Model file for the job. Use its own axes, mm. A direction names the side the tool comes from. Give positions to 0.01 mm unless a question says otherwise; leave off trailing zeros. Order: outer loops, then holes, each group sorted by start corner. A loop starts at its lowest first (then second) coordinate and runs counter-clockwise, first axis right, second up. Notation, with made-up numbers: (51, 9.5) - (75, 9.5) arc R26 ccw to (75, 40.5) - close; hole circle Ø4 at (68, 28.25). An arc over 180 degrees is marked (long way). Return JSON: item names as keys, results as strings. Group by question number.
from build123d import *

# Parameters (mm, degrees)
F0_W      = 50.8
F0_H      = 50.8
F1_DEPTH  = 50.8
F2_W      = 38.1
F2_H      = 38.1
F3_DEPTH  = 1.27
F4_W      = 38.1
F4_H      = 38.1
F5_DEPTH  = 1.27
F6_W      = 38.1
F6_H      = 38.1
F7_DEPTH  = 1.27
F8_W      = 38.1
F8_H      = 38.1
F9_DEPTH  = 1.27
F10_W     = 8.382
F10_H     = 8.382
F11_DEPTH = 12.7
F13_DEPTH = 25.4
F14_SIZE  = 25.39999


# Not quite as in the source:
# - a fillet or chamfer is up to 0.001 mm smaller than in the source, because OpenCascade refuses the exact size


with BuildPart() as f1:
    # F0 (on Top) → F1 (new body)
    with BuildSketch(Plane.XY):
        Rectangle(F0_W, F0_H)
    extrude(amount=F1_DEPTH)

    # F2 (on face) → F3 (cut)
    with BuildSketch(Plane.XZ.offset(25.4)):
        with Locations((0, 25.4)):
            Rectangle(F2_W, F2_H)
        with BuildLine():
            Line((-12.9850329568, 8.9432131499), (-12.9850329568, 42.6816119349))
            Line((-12.9850329568, 42.6816119349), (-2.484703985, 42.6816119349))
            add(Edge.make_bspline(
                [(-2.484703985, 42.6816119349), (4.6927360717, 42.6816119349), (7.9343988133, 40.6398813015)],
                knots=[0, 0, 0, 1, 1, 1], degree=2))
            add(Edge.make_bspline(
                [(7.9343988133, 40.6398813015), (11.176061555, 38.5981506681), (11.176061555, 34.1454795218)],
                knots=[0, 0, 0, 1, 1, 1], degree=2))
            add(Edge.make_bspline(
                [(11.176061555, 34.1454795218), (11.176061555, 31.1179585102), (9.7582956179, 29.1796066431)],
                knots=[0, 0, 0, 1, 1, 1], degree=2))
            add(Edge.make_bspline(
                [(9.7582956179, 29.1796066431), (8.3405296807, 27.2412547759), (5.9849706498, 26.8498923037)],
                knots=[0, 0, 0, 1, 1, 1], degree=2))
            Line((5.9849706498, 26.8498923037), (5.9849706498, 26.6209821784))
            add(Edge.make_bspline(
                [(5.9849706498, 26.6209821784), (9.1897124035, 25.9047150123), (10.6111704394, 23.9442105523)],
                knots=[0, 0, 0, 1, 1, 1], degree=2))
            add(Edge.make_bspline(
                [(10.6111704394, 23.9442105523), (12.0326284753, 21.9837060924), (12.0326284753, 18.7272749556)],
                knots=[0, 0, 0, 1, 1, 1], degree=2))
            add(Edge.make_bspline(
                [(12.0326284753, 18.7272749556), (12.0326284753, 14.1121514623), (8.694971165, 11.5276823061)],
                knots=[0, 0, 0, 1, 1, 1], degree=2))
            add(Edge.make_bspline(
                [(8.694971165, 11.5276823061), (5.3573138547, 8.9432131499), (-0.3654392769, 8.9432131499)],
                knots=[0, 0, 0, 1, 1, 1], degree=2))
            Line((-0.3654392769, 8.9432131499), (-12.9850329568, 8.9432131499))
        make_face(mode=Mode.SUBTRACT)
        with BuildLine():
            Line((-5.8297454929, 36.8185590491), (-5.8297454929, 29.3162142985))
            Line((-5.8297454929, 29.3162142985), (-1.6798264478, 29.3162142985))
            add(Edge.make_bspline(
                [(-1.6798264478, 29.3162142985), (1.2295474023, 29.3162142985), (2.5328582768, 30.2170864044)],
                knots=[0, 0, 0, 1, 1, 1], degree=2))
            add(Edge.make_bspline(
                [(2.5328582768, 30.2170864044), (3.8361691513, 31.1179585102), (3.8361691513, 33.1929180328)],
                knots=[0, 0, 0, 1, 1, 1], degree=2))
            add(Edge.make_bspline(
                [(3.8361691513, 33.1929180328), (3.8361691513, 35.1349619988), (2.4184032142, 35.9767605239)],
                knots=[0, 0, 0, 1, 1, 1], degree=2))
            add(Edge.make_bspline(
                [(2.4184032142, 35.9767605239), (1.0006372771, 36.8185590491), (-2.07118892, 36.8185590491)],
                knots=[0, 0, 0, 1, 1, 1], degree=2))
            Line((-2.07118892, 36.8185590491), (-5.8297454929, 36.8185590491))
        make_face()
        with BuildLine():
            Line((-1.3992269394, 23.64515055), (-5.8297454929, 23.64515055))
            Line((-5.8297454929, 23.64515055), (-5.8297454929, 14.8505712213))
            Line((-5.8297454929, 14.8505712213), (-1.1703168141, 14.8505712213))
            add(Edge.make_bspline(
                [(-1.1703168141, 14.8505712213), (1.7833622215, 14.8505712213), (3.1900518623, 15.9803534524)],
                knots=[0, 0, 0, 1, 1, 1], degree=2))
            add(Edge.make_bspline(
                [(3.1900518623, 15.9803534524), (4.596741503, 17.1101356836), (4.596741503, 19.4435421217)],
                knots=[0, 0, 0, 1, 1, 1], degree=2))
            add(Edge.make_bspline(
                [(4.596741503, 19.4435421217), (4.596741503, 23.64515055), (-1.3992269394, 23.64515055)],
                knots=[0, 0, 0, 1, 1, 1], degree=2))
        make_face()
    extrude(amount=-F3_DEPTH, mode=Mode.SUBTRACT)

    # F4 (on face) → F5 (cut)
    with BuildSketch(Plane.YZ.offset(25.4)):
        with Locations((0, 25.4)):
            Rectangle(F4_W, F4_H)
        with BuildLine():
            Line((8.2110515278, 41.6381866004), (15.0563287647, 41.6381866004))
            Line((15.0563287647, 41.6381866004), (15.0563287647, 20.6913548071))
            add(Edge.make_bspline(
                [(15.0563287647, 20.6913548071), (15.0563287647, 17.098647189), (13.4513025803, 14.3988018192)],
                knots=[0, 0, 0, 1, 1, 1], degree=2))
            add(Edge.make_bspline(
                [(13.4513025803, 14.3988018192), (11.8462763959, 11.6989564493), (8.8098361308, 10.2569130563)],
                knots=[0, 0, 0, 1, 1, 1], degree=2))
            add(Edge.make_bspline(
                [(8.8098361308, 10.2569130563), (5.7733958658, 8.8148696632), (1.6350502071, 8.8148696632)],
                knots=[0, 0, 0, 1, 1, 1], degree=2))
            add(Edge.make_bspline(
                [(1.6350502071, 8.8148696632), (-4.6078993227, 8.8148696632), (-8.0624258786, 12.0178358237)],
                knots=[0, 0, 0, 1, 1, 1], degree=2))
            add(Edge.make_bspline(
                [(-8.0624258786, 12.0178358237), (-11.5169524345, 15.2208019843), (-11.5169524345, 20.776389307)],
                knots=[0, 0, 0, 1, 1, 1], degree=2))
            Line((-11.5169524345, 20.776389307), (-11.5169524345, 41.6381866004))
            Line((-11.5169524345, 41.6381866004), (-4.6787614059, 41.6381866004))
            Line((-4.6787614059, 41.6381866004), (-4.6787614059, 21.81806193))
            add(Edge.make_bspline(
                [(-4.6787614059, 21.81806193), (-4.6787614059, 18.0765439371), (-3.1729421379, 16.3262504822)],
                knots=[0, 0, 0, 1, 1, 1], degree=2))
            add(Edge.make_bspline(
                [(-3.1729421379, 16.3262504822), (-1.66712287, 14.5759570272), (1.8122054151, 14.5759570272)],
                knots=[0, 0, 0, 1, 1, 1], degree=2))
            add(Edge.make_bspline(
                [(1.8122054151, 14.5759570272), (5.178154367, 14.5759570272), (6.6946029474, 16.3368797946)],
                knots=[0, 0, 0, 1, 1, 1], degree=2))
            add(Edge.make_bspline(
                [(6.6946029474, 16.3368797946), (8.2110515278, 18.0978025621), (8.2110515278, 21.8605791799)],
                knots=[0, 0, 0, 1, 1, 1], degree=2))
            Line((8.2110515278, 21.8605791799), (8.2110515278, 41.6381866004))
        make_face(mode=Mode.SUBTRACT)
    extrude(amount=-F5_DEPTH, mode=Mode.SUBTRACT)

    # F6 (on face) → F7 (cut)
    with BuildSketch(Plane(origin=(0, 25.4, 0), x_dir=(-1, 0, 0), z_dir=(0, 1, 0))):
        with Locations((0, 25.4)):
            Rectangle(F6_W, F6_H)
        Polygon((-0.3206622132, 36.6013397979), (-0.3206622132, 8.6884368211), (-7.5084387172, 8.6884368211), (-7.5084387172, 36.6013397979), (-16.713836696, 36.6013397979), (-16.713836696, 42.5800269622), (8.8773180396, 42.5800269622), (8.8773180396, 36.6013397979), align=None, mode=Mode.SUBTRACT)
    extrude(amount=-F7_DEPTH, mode=Mode.SUBTRACT)

    # F8 (on face) → F9 (cut)
    with BuildSketch(Plane(origin=(-25.4, 0, 0), x_dir=(0, -1, 0), z_dir=(-1, 0, 0))):
        with Locations((0, 25.4)):
            Rectangle(F8_W, F8_H)
        Polygon((0.4234320166, 35.945847888), (0.4234320166, 10.2160740644), (-6.2021727762, 10.2160740644), (-6.2021727762, 35.945847888), (-14.6875964581, 35.945847888), (-14.6875964581, 41.4569288611), (8.902018129, 41.4569288611), (8.902018129, 35.945847888), align=None, mode=Mode.SUBTRACT)
    extrude(amount=-F9_DEPTH, mode=Mode.SUBTRACT)

    # F10 (on face) → F11 (join)
    with BuildSketch(Plane.XY.offset(50.8)):
        Rectangle(F10_W, F10_H)
    extrude(amount=F11_DEPTH)

    # F12 (on face) → F13 (join)
    with BuildSketch(Plane(origin=(0, 0, 0), x_dir=(1, 0, 0), z_dir=(0, 0, -1))):
        with BuildLine():
            ThreePointArc((3.01e-08, -25.4), (17.9605122528, -17.9605122315), (25.4, 0))
            ThreePointArc((25.4, 0), (17.9605122594, 17.9605122249), (4.89e-08, 25.4))
            ThreePointArc((4.89e-08, 25.4), (-17.9605122127, 17.9605122716), (-25.4, 3.44e-08))
            ThreePointArc((-25.4, 3.44e-08), (-17.9605122437, -17.9605122406), (3.01e-08, -25.4))
        make_face()
    extrude(amount=F13_DEPTH)

    # F14 (size 25.4 in the source; OpenCascade refuses exactly that, so slightly less here)
    f14_edges = [f1.edges().sort_by_distance(p)[0] for p in [
        (0, -25.4, -25.4),
    ]]
    chamfer(f14_edges, length=F14_SIZE)


solid = f1.part
(1) Drop flat-ended pins along their axis: pin 1 Ø10 at (x, y) = (-1.5, -15.5) entering from -Z; pin 2 Ø6 at (x, y) = (5.5, -12) entering from -Z; pin 3 Ø20.5 at (x, y) = (-9.5, -18) entering from -Z. Give the stop position or say it passes through.
(2) 3-axis set-ups, long thin cutter, end or side, ignore diameter. For faces 5 (the face through (0, 4.191, 57)), 6 (the face through (-4.191, 0, 57)), 7 (the face through (-20, -19, 0)), 8 (the face through (20, -20, 0)), 9 (the face through (19, 20, 0)): which of +Z, -Z, +X, -X, +Y, -Y reach the whole face in a straight line?
(3) Drill centre lines: L1, parallel to Y at x = -17, z = 13.5; L2, parallel to X at y = -3.5, z = 56.5; L3, parallel to X at y = 4, z = 23. Where is each one in solid material? Low to high.
(4) Slice it at B-B (z = -7). Give the cut face in (x, y), and give its area (3 significant figures).
(5) Slice it at A-A (z = 52). Give the cut face in (x, y), and give its area (3 significant figures).
(6) Pull direction X, two halves, no side cores. Call faces 1 (the face through (4.191, 0, 57)), 2 (the face through (12, -24.13, 26)), 3 (the face through (-1, -24.13, 19)), 4 (the face through (0, -4.191, 57)): released by +X, released by -X, zero draft, split by the parting line, or undercut.
Result set:
{
 "1": {"pin 1": "stops at z = -14.83", "pin 2": "stops at z = -15.2", "pin 3": "stops at z = -15.3"},
 "2": {"face 5": "+Z, +X, -X, +Y", "face 6": "+Z, -X, +Y, -Y", "face 7": "-Z, -X, -Y", "face 8": "-Z, +X, -Y", "face 9": "-Z, +X, +Y"},
 "3": {"L1": "y = -24.13 to 24.13", "L2": "x = -4.19 to 4.19", "L3": "x = -25.4 to 24.13"},
 "4": {"outline": "circle Ø36.8 at (0, 0)", "area": "1,060 mm²"},
 "5": {"outline": "(-4.19, -4.19) - (4.19, -4.19) - (4.19, 4.19) - (-4.19, 4.19) - close", "area": "70.3 mm²"},
 "6": {"face 1": "released by +X", "face 2": "undercut", "face 3": "undercut", "face 4": "zero draft"}
}
